Autodesk Inventor part; units mm, degrees
ref_plane "YZ Plane" through (0, 0, 0) normal (1, 0, 0) x (0, 1, 0)
ref_plane "XZ Plane" through (0, 0, 0) normal (0, 1, 0) x (-1, 0, 0)
sketch "Skizze1" plane through (0, 0, 0) normal (0, 1, 0) x (-1, 0, 0)
  circle A0 centre (0, 0) radius 30
  dimension "d0" = 60
extrude "Extrusion1" add sketch "Skizze1" along normal mid plane 3
sketch "Skizze2" plane through (0, 1.5, 0) normal (0, 1, 0) x (1, 0, 0)
  line L0 (0, 43.5645) -> (0, -46.3445) construction
  circle A0 centre (0, 17.5) radius 8
  circle A1 centre (-16.6435, 5.4078) radius 8
  circle A2 centre (-10.2862, -14.1578) radius 8
  circle A3 centre (10.2862, -14.1578) radius 8
  circle A4 centre (16.6435, 5.4078) radius 8
  point P0 (0, 0)
  dimension "d3" = 16
  dimension "d4" = 17.5
  dimension "d7" = 360
extrude "Extrusion2" cut sketch "Skizze2" against normal through all
sketch "Skizze3" plane through (0, 1.5, 0) normal (0, 1, 0) x (1, 0, 0)
  point P0 (0, 0)
  point P1 (0, 0)
hole "Bohrung1" at (0, 1.5, 0) direction (0, -1, 0) diameter 4.917 end through all
ref_plane "Arbeitsebene1" through (0, 0, -30) normal (0, 0, 1) x (1, 0, 0)
sketch "Skizze4" plane through (0, 0, -30) normal (0, 0, 1) x (1, 0, 0)
  point P0 (0, 0)
  point P1 (0, 0)
hole "Bohrung2" at (0, 0, -30) direction (0, 0, 1) diameter 1.567 depth 6.3 tip angle 118
pattern_circular "Runde Anordnung1" count 3 over 360 about axis through (0, -10, 0) along (0, 1, 0) of "Bohrung2"
properties part number "Ronde_Engine"
Design review of the part built by this model. Coordinates are the model's own, in mm. A direction names the side the tool comes from. Round coordinates to 2 decimals unless told otherwise and drop trailing zeros. Write each loop counter-clockwise with the first axis right and the second up, starting at its lowest first coordinate (ties: lowest second). Pieces come first, ordered by that corner, then holes. Notation, with made-up numbers: M 87.25,-21 L 140.25,-21 A19 cw 140.25,14 Z; hole C 70.25,57.5 d7. An arc over 180 degrees is marked long. One line per item, written item: value. Start each with the question number.
1. To check wall thickness, follow probe 1 along Z at (x, y) = (17, 1.1); probe 2 along Z at (x, y) = (-12, 0.5); probe 3 along X at (y, z) = (-0.15, 1). State the ranges of each line that lie inside material, in increasing order. Write a range as from..to.
2. Take a section at A-A on x = 0. State the section outline as (y, z) points, then the cut area to 3 significant figures.
3. Take a section at C-C on x = 19. State the section outline as (y, z) points.
4. Take a section at B-B on z = -17.5. State the section outline as (x, y) points, then the cut area to 3 significant figures.
5. For faces 1 (the face through (-0.738, -0.021, 2.345)), 2 (the face through (-0.235, 0.747, -27.699)), 3 (the face through (20.17, 0.13, 11.69)), list the 3-axis set-ups (+Z, -Z, +X, -X, +Y, -Y) from which the entire face can be reached by the end or side of a thin tool; tool diameter is ignored.
6. Take a section at D-D on z = 0. State the section outline as (x, y) points, then the cut area to 3 significant figures.
7. Draft analysis for pull direction Z (two halves, no side actions). For faces 4 (the face through (-20.162, 0.126, 11.701)), 5 (the face through (29.97, -0.02, -1.32)), 6 (the face through (0, 1.5, -6)), state which applies: pulls with the +Z half, pulls with the -Z half, needs draft (parallel to the pull), parting line crosses it, or undercut.
8. Clearance check with flat-ended pins moving along their axes: P1, Ø14.5, axis at x = -10.29, z = 14.16, coming from the +Y side; P2, Ø1, axis at x = -16.5, y = 1, coming from the -Z side; P3, Ø1.4, axis at x = 0, y = 0, coming from the -Z side. State where each tip first meets the part, or that it passes through.
Computed:
1. probe 1: z = -24.72..-13.4, 2.58..9.81, 18.51..24.72
1. probe 2: z = -27.5..-11.92, 1.11..6.34, 21.97..27.5
1. probe 3: x = -29.98..-21.43, -11.85..-2.25, 2.25..11.85, 21.43..29.98
2. outline: M -1.5,-30 L -0.78,-30 L -0.78,-25.5 L -1.5,-25.5 Z; M -1.5,-9.5 L 1.5,-9.5 L 1.5,-2.46 L -1.5,-2.46 Z; M -1.5,2.46 L 1.5,2.46 L 1.5,30 L -1.5,30 Z; M 0.78,-30 L 1.5,-30 L 1.5,-25.5 L 0.78,-25.5 Z
2. area: 110 mm²
3. outline: M -1.5,-23.22 L 1.5,-23.22 L 1.5,-13.05 L -1.5,-13.05 Z; M -1.5,2.24 L 1.5,2.24 L 1.5,23.22 L -1.5,23.22 Z
4. outline: M -24.37,-1.5 L -8,-1.5 L -8,1.5 L -24.37,1.5 Z; M 8,-1.5 L 24.37,-1.5 L 24.37,1.5 L 8,1.5 Z
4. area: 98.2 mm²
5. face 1: +Y, -Y
5. face 2: -Z
5. face 3: none
6. outline: M -30,-1.5 L -22.54,-1.5 L -22.54,1.5 L -30,1.5 Z; M -10.75,-1.5 L -2.46,-1.5 L -2.46,1.5 L -10.75,1.5 Z; M 2.46,-1.5 L 10.75,-1.5 L 10.75,1.5 L 2.46,1.5 Z; M 22.54,-1.5 L 30,-1.5 L 30,1.5 L 22.54,1.5 Z
6. area: 94.5 mm²
7. face 4: undercut
7. face 5: parting line crosses it
7. face 6: needs draft
8. P1: passes through
8. P2: stops at z = -25.38
8. P3: stops at z = -9.53
